The model under review builds one solid part; all positions refer to its coordinate system, in mm. Face numbers are marked on the shaded views. A direction names the side the tool comes from. Coordinates: 2 decimals unless noted, no trailing zeros. Loops run counter-clockwise (first coordinate to the right, second up) from the corner with the lowest first, then second, coordinate; pieces in that order, holes last. Notation, with made-up numbers: (69, 49) - (119, 49) arc R20 cw to (119, 70) - close; hole circle Ø10 at (81.25, 21.5). An arc over 180 degrees is marked (long way). Use a Markdown table: item, result. Add a question column.
1) The part is to be moulded in two halves that separate along Z. For the marked faces 3, 4 and 5, say which applies: pulls with the +Z half, pulls with the -Z half, needs draft (parallel to the pull), parting line crosses it, or undercut.
2) To check wall thickness, follow L1, parallel to Z at x = 11, y = 0 (3 decimals); L2, parallel to X at y = -2, z = 7; L3, parallel to Z at x = 5, y = -5.5. State the ranges of each line that lie inside material, in increasing order. Write a range as [from, to].
3) Clearance check with flat-ended pins moving along their axes: pin 1 (8 mm diameter, centred on x = 15, z = 4.5, fed in from -Y); pin 2 (6 mm diameter, centred on x = 8.5, z = -3.5, fed in from +Y); pin 3 (1.5 mm diameter, centred on x = 4, y = -2.5, fed in from +Z). State where each tip first meets the part, or that it passes through.
4) For the marked faces 1 and 2, list the 3-axis set-ups (+Z, -Z, +X, -X, +Y, -Y) from which the entire face can be reached by the end or side of a thin tool; tool diameter is ignored.
5) Add section C-C, the plane x = 11.5. Give the boundary of the cut face in (y, z) (3 decimals).
```python
from build123d import *


with BuildPart() as part:
    # Sketch1 → BaseBody (revolve)
    with BuildSketch(Plane.XY):
        with BuildLine():
            Line((0, 3.9624), (0, 7.4676))
            ThreePointArc((0, 7.4676), (0.23062412, 8.02437588), (0.7874, 8.255))
            Line((0.7874, 8.255), (3.9624, 8.255))
            Line((3.9624, 8.255), (3.9624, 6.6675))
            ThreePointArc((3.9624, 6.6675), (3.737893597, 6.125493597), (4.2799, 6.35))
            Line((4.2799, 6.35), (16.3449, 6.35))
            Line((16.3449, 6.35), (16.6624, 6.0325))
            Line((16.6624, 6.0325), (16.6624, 3.175))
            Line((16.6624, 3.175), (0.7874, 3.175))
            ThreePointArc((0.7874, 3.175), (0.23062412, 3.40562412), (0, 3.9624))
        make_face()
    revolve(axis=Axis((0, 0, 0), (1, 0, 0)))


solid = part.part
```
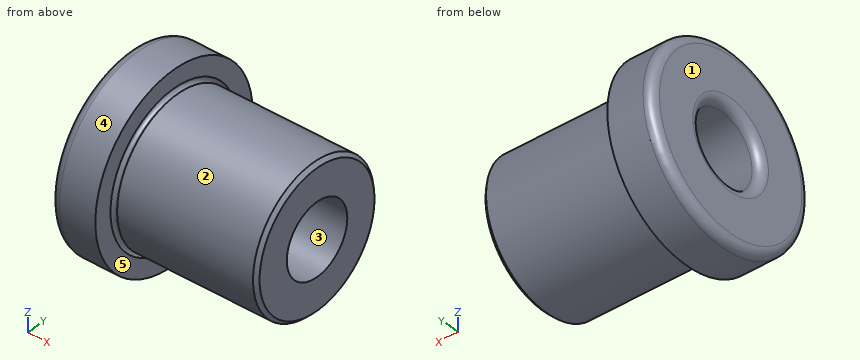
From the geometry:
| question | item | result |
|---|---|---|
| 1 | face 3 | undercut |
| 1 | face 4 | parting line crosses it |
| 1 | face 5 | needs draft |
| 2 | L1 | z = [-6.35, -3.175], [3.175, 6.35] |
| 2 | L2 | x = [0, 3.96] |
| 2 | L3 | z = [-3.17, 3.17] |
| 3 | pin 1 | stops at y = -6.33 |
| 3 | pin 2 | stops at y = 6.33 |
| 3 | pin 3 | stops at z = 8.07 |
| 4 | face 1 | +Z, -Z, -X, +Y, -Y |
| 4 | face 2 | +X |
| 5 | outline | circle Ø12.7 at (0, 0); hole circle Ø6.35 at (0, 0) |
